The listing builds one solid part. Answer for the finished solid, in the listing's coordinates (mm). Face numbers are marked on the shaded views. Coordinates: 2 decimals unless noted, no trailing zeros. Loops run counter-clockwise (first coordinate to the right, second up) from the corner with the lowest first, then second, coordinate; pieces in that order, holes last. Notation, with made-up numbers: M 61.25,69 L 80.25,69 A28 ccw 80.25,95 Z; hole C 14,47 d2. An arc over 180 degrees is marked long. Answer as a JSON object with one key per item and string values. Group by question number.
1. Given pin 1 (2.5 mm diameter, centred on x = 0, z = 25.4, fed in from +Y); pin 2 (1 mm diameter, centred on y = 3, z = -9, fed in from +X); pin 3 (1 mm diameter, centred on y = 4.5, z = 11, fed in from +X) (3 decimals); pin 4 (3 mm diameter, centred on x = -6, y = 3.5, fed in from +Z), each flat-ended and moving along its own axis, determine where each tip first touches the part or whether it passes through.
2. A cutting plane is placed at D-D on y = 2.75. State how many separate pieces and enclosed holes the cut face has, and give its area (3 significant figures).
3. Straight lines are drawn through the part: L1, parallel to X at y = 1.5, z = 3.5; L2, parallel to Z at x = -5.25, y = 5.75; L3, parallel to X at y = 5.25, z = 0. For each, find the intervals that lie inside material, in ascending order.
4. Determine the mould class of the marked faces 1, 2 and 3 for opening direction X: released by +X, released by -X, zero draft, split by the parting line, or undercut.
5. A cutting plane is placed at C-C on x = 4.5. Give the vertices of the cut face in (y, z), and give its area (3 significant figures).
6. A cutting plane is placed at A-A on z = 0. Give the vertices of the cut face in (x, y).
7. A cutting plane is placed at B-B on x = 0. Give the vertices of the cut face in (y, z), and give its area (3 significant figures).
from build123d import *

# Parameters (mm, degrees)
SKETCH1_R                      = 3.81
BOSS_EXTRUDE1_DEPTH            = 6.35
F_6_32_TAPPED_HOLE1_D          = 2.7051
F_6_CLEARANCE_HOLE1_AT_2_COUNT = 2
F_6_CLEARANCE_HOLE1_AT_2_PITCH = 7.48452257
F_6_CLEARANCE_HOLE1_AT_3_COUNT = 2
F_6_CLEARANCE_HOLE1_AT_3_PITCH = 19.558
F_6_CLEARANCE_HOLE1_AT_4_COUNT = 2
F_6_CLEARANCE_HOLE1_AT_4_PITCH = 18.069235897
CIRPATTERN1_COUNT              = 2
CIRPATTERN1_ANGLE              = 90


with BuildPart() as part:
    # Sketch1 → Boss-Extrude1 (new body)
    with BuildSketch(Plane(origin=(0, 0, 0), x_dir=(1, 0, 0), z_dir=(0, 1, 0))):
        with BuildLine():
            Line((-12.474760456, 2.38125), (-7.796725285, 26.88828125))
            ThreePointArc((-7.796725285, 26.88828125), (0, 33.3375), (7.796725285, 26.88828125))
            Line((7.796725285, 26.88828125), (12.474760456, 2.38125))
            ThreePointArc((12.474760456, 2.38125), (12.7, 0), (12.474760456, -2.38125))
            Line((12.474760456, -2.38125), (7.796725285, -26.88828125))
            ThreePointArc((7.796725285, -26.88828125), (0, -33.3375), (-7.796725285, -26.88828125))
            Line((-7.796725285, -26.88828125), (-12.474760456, -2.38125))
            ThreePointArc((-12.474760456, -2.38125), (-12.7, 0), (-12.474760456, 2.38125))
        make_face()
        Circle(SKETCH1_R, mode=Mode.SUBTRACT)
    extrude(amount=BOSS_EXTRUDE1_DEPTH)

    # #6-32 Tapped Hole1 (through all)
    with Locations(Plane(origin=(0, 6.35, 0), x_dir=(1, 0, 0), z_dir=(0, 1, 0))):
        with Locations((0, -25.4), (0, 25.4)):
            Hole(F_6_32_TAPPED_HOLE1_D / 2)

    # Sketch6 → #6 Clearance Hole1 (revolve, cut)
    with BuildSketch(Plane(origin=(-3.742261285, 6.35, -9.034617948), x_dir=(0, 0, 1), z_dir=(1, 0, 0))):
        Polygon((0, 0), (0, 10.538824014), (1.89865, 9.398), (1.89865, 0), align=None)
    f_6_clearance_hole1 = revolve(axis=Axis((-3.742261285, 12.7, -9.034617948), (0, -1, 0)), mode=Mode.SUBTRACT)

    # #6 Clearance Hole1 at 2: #6 Clearance Hole1 ×2
    with Locations(*[(i * F_6_CLEARANCE_HOLE1_AT_2_PITCH, 0, 0) for i in range(1, F_6_CLEARANCE_HOLE1_AT_2_COUNT)]):
        add(f_6_clearance_hole1, mode=Mode.SUBTRACT)

    # #6 Clearance Hole1 at 3: #6 Clearance Hole1 ×2
    with Locations(*[Vector(0.382683432, 0, 0.923879533) * (i * F_6_CLEARANCE_HOLE1_AT_3_PITCH) for i in range(1, F_6_CLEARANCE_HOLE1_AT_3_COUNT)]):
        add(f_6_clearance_hole1, mode=Mode.SUBTRACT)

    # #6 Clearance Hole1 at 4: #6 Clearance Hole1 ×2
    with Locations(*[(0, 0, i * F_6_CLEARANCE_HOLE1_AT_4_PITCH) for i in range(1, F_6_CLEARANCE_HOLE1_AT_4_COUNT)]):
        add(f_6_clearance_hole1, mode=Mode.SUBTRACT)

    # CirPattern1: #6 Clearance Hole1 ×2 about axis
    cirpattern1_axis = Axis((0, 0, 0), (0, 1, 0))
    for i in range(1, CIRPATTERN1_COUNT):
        add(f_6_clearance_hole1.rotate(cirpattern1_axis, i * CIRPATTERN1_ANGLE / (CIRPATTERN1_COUNT - 1)), mode=Mode.SUBTRACT)

    # CirPattern1 copy 1 sketch → CirPattern1 copy 1 (revolve, cut)
    with BuildSketch(Plane(origin=(-9.034617948, 6.35, -3.742261285), x_dir=(1, 0, 0), z_dir=(0, 0, -1))):
        Polygon((0, 0), (0, 10.538824014), (1.89865, 9.398), (1.89865, 0), align=None)
    revolve(axis=Axis((-9.034617948, 12.7, -3.742261285), (0, -1, 0)), mode=Mode.SUBTRACT)

    # CirPattern1 copy 2 sketch → CirPattern1 copy 2 (revolve, cut)
    with BuildSketch(Plane(origin=(9.034617948, 6.35, -3.742261285), x_dir=(1, 0, 0), z_dir=(0, 0, -1))):
        Polygon((0, 0), (0, 10.538824014), (1.89865, 9.398), (1.89865, 0), align=None)
    revolve(axis=Axis((9.034617948, 12.7, -3.742261285), (0, -1, 0)), mode=Mode.SUBTRACT)

    # CirPattern1 copy 3 sketch → CirPattern1 copy 3 (revolve, cut)
    with BuildSketch(Plane(origin=(9.034617948, 6.35, 3.742261285), x_dir=(1, 0, 0), z_dir=(0, 0, -1))):
        Polygon((0, 0), (0, 10.538824014), (1.89865, 9.398), (1.89865, 0), align=None)
    revolve(axis=Axis((9.034617948, 12.7, 3.742261285), (0, -1, 0)), mode=Mode.SUBTRACT)


solid = part.part
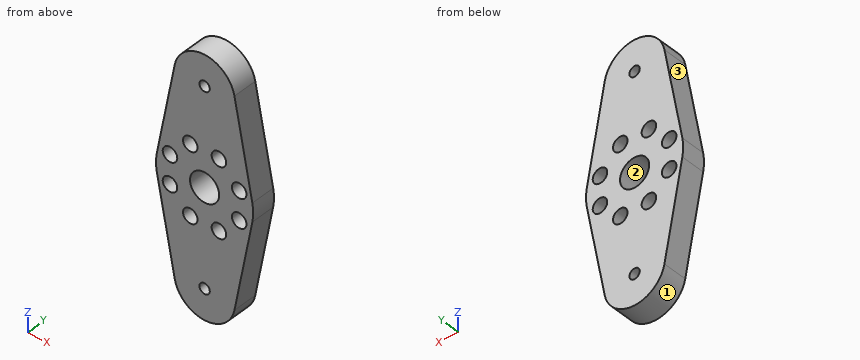
From the geometry:
{
 "1": {"pin 1": "passes through", "pin 2": "stops at x = 11.31", "pin 3": "stops at x = 10.925", "pin 4": "stops at z = 31.94"},
 "2": {"separate pieces": "1", "enclosed holes": "11", "area": "1,120 mm²"},
 "3": {"L1": "x = -12.26 to -10.92, -7.15 to -1.51, 1.51 to 7.15, 10.92 to 12.26", "L2": "z = -31.35 to -10.19, -7.88 to 7.88, 10.19 to 31.35", "L3": "x = -12.7 to -3.81, 3.81 to 12.7"},
 "4": {"face 1": "split by the parting line", "face 2": "undercut", "face 3": "released by -X"},
 "5": {"outline": "M 0,-31.94 L 6.35,-31.94 L 6.35,-10.78 L 0,-10.78 Z; M 0,-7.29 L 6.35,-7.29 L 6.35,7.29 L 0,7.29 Z; M 0,10.78 L 6.35,10.78 L 6.35,31.94 L 0,31.94 Z", "area": "361 mm²"},
 "6": {"outline": "M -12.7,0 L -3.81,0 L -3.81,6.35 L -12.7,6.35 Z; M 3.81,0 L 12.7,0 L 12.7,6.35 L 3.81,6.35 Z"},
 "7": {"outline": "M 0,-33.34 L 6.35,-33.34 L 6.35,-26.75 L 0,-26.75 Z; M 0,-24.05 L 6.35,-24.05 L 6.35,-3.81 L 0,-3.81 Z; M 0,3.81 L 6.35,3.81 L 6.35,24.05 L 0,24.05 Z; M 0,26.75 L 6.35,26.75 L 6.35,33.34 L 0,33.34 Z", "area": "341 mm²"}
}
